```python
from build123d import *

# Parameters (mm, degrees)
BOSS_EXTRUDE1_DEPTH       = 3.175
SKETCH3_R                 = 5.55625
CUT_EXTRUDE1_DEPTH        = 31.120694713
SKETCH4_W                 = 31.75
SKETCH4_H                 = 3.175
BOSS_EXTRUDE2_DEPTH       = 12.7
SKETCH5_R                 = 1.5875
CUT_EXTRUDE2_DEPTH        = 45.22263278
F_2_0MM_DOWEL_HOLE1_D     = 2
F_2_0MM_DOWEL_HOLE1_DEPTH = 12.7
F_2_0MM_DOWEL_HOLE1_TIP   = 0.600860619


with BuildPart() as part:
    # Sketch1 → Boss-Extrude1 (new body)
    with BuildSketch(Plane.XY):
        with BuildLine():
            ThreePointArc((15.875, 0), (0, 15.875), (-15.875, 0))
            Line((-15.875, 0), (15.875, 0))
        make_face()
        with BuildLine():
            ThreePointArc((15.875, 0), (0, -15.875), (-15.875, 0))
            Line((-15.875, 0), (-15.875, -25.4))
            Line((-15.875, -25.4), (15.875, -25.4))
            Line((15.875, -25.4), (15.875, 0))
        make_face()
        with BuildLine():
            Line((15.875, 0), (-15.875, 0))
            ThreePointArc((-15.875, 0), (0, -15.875), (15.875, 0))
        make_face()
    extrude(amount=BOSS_EXTRUDE1_DEPTH)

    # Sketch3 → Cut-Extrude1 (cut, through all)
    with BuildSketch(Plane.XY.offset(3.175)):
        Circle(SKETCH3_R)
    extrude(amount=-CUT_EXTRUDE1_DEPTH, mode=Mode.SUBTRACT)

    # Sketch4 → Boss-Extrude2 (add)
    with BuildSketch(Plane.XY.offset(3.175)):
        with Locations((0, -23.8125)):
            Rectangle(SKETCH4_W, SKETCH4_H)
    extrude(amount=BOSS_EXTRUDE2_DEPTH)

    # Sketch5 → Cut-Extrude2 (cut, through all)
    with BuildSketch(Plane(origin=(0, -22.225, 0), x_dir=(1, 0, 0), z_dir=(0, 1, 0))):
        with Locations(Location((-9.525, -9.525, 0), (0, 0, 270))):
            Circle(SKETCH5_R)
        with Locations(Location((9.525, -9.525, 0), (0, 0, 90))):
            Circle(SKETCH5_R)
    extrude(amount=-CUT_EXTRUDE2_DEPTH, mode=Mode.SUBTRACT)

    # Ø2.0mm Dowel Hole1
    with Locations(Plane.XY.offset(3.175)):
        with Locations((-8.001, 0), (8.001, 0)):
            Hole(F_2_0MM_DOWEL_HOLE1_D / 2, depth=F_2_0MM_DOWEL_HOLE1_DEPTH)
            with Locations((0, 0, -(F_2_0MM_DOWEL_HOLE1_DEPTH + F_2_0MM_DOWEL_HOLE1_TIP / 2))):  # 118° drill point
                Cone(0, F_2_0MM_DOWEL_HOLE1_D / 2, F_2_0MM_DOWEL_HOLE1_TIP, mode=Mode.SUBTRACT)


solid = part.part
```
Here's how the part is built. I have some questions about the finished solid (model axes, mm). A direction names the side the tool comes from. Coordinates: 2 decimals unless noted, no trailing zeros. Order: outer loops, then holes, each group sorted by start corner. A loop starts at its lowest first (then second) coordinate and runs counter-clockwise, first axis right, second up.
Item 1: I need wall thicknesses on probe 1 along Y at (x, z) = (3, 5.5) (3 decimals); probe 2 along Z at (x, y) = (5, -6) (3 decimals); probe 3 along Y at (x, z) = (0.5, 2). Which ranges of each line are inside material? Lowest first, please.
Response values:
probe 1: y = -25.4 to -22.225
probe 2: z = 0 to 3.175
probe 3: y = -25.4 to -5.53, 5.53 to 15.87
Item 2: Which directions (+Z, -Z, +X, -X, +Y, -Y) give clear straight access to the entire face, cutting with the end or side of a thin tool? Please do faces 4 (the face through (0, -22.225, 9)), 5 (the face through (15.875, -16, 3)).
Response values:
face 4: +Z, +X, -X, +Y
face 5: +Z, -Z, +X, +Y, -Y
Item 3: Thinking about a two-plate mould opening in Y: for faces 1 (the face through (0, -25.4, 8)), 2 (the face through (8.8, -0.6, 1.6)), 3 (the face through (0, -24, 15.875)), which applies, pulls with the +Y half, pulls with the -Y half, needs draft (parallel to the pull), parting line crosses it, or undercut?
Response values:
face 1: pulls with the -Y half
face 2: undercut
face 3: needs draft
Item 4: If we section it at D-D, the plane y = 4: List the corners of the cut face in (x, z) for me (3 decimals), then the cut area to 3 significant figures.
Response values:
outline: (-15.363, 0) - (-3.856, 0) - (-3.856, 3.175) - (-15.363, 3.175) - close; (3.856, 0) - (15.363, 0) - (15.363, 3.175) - (3.856, 3.175) - close
area: 73.1 mm2
Item 5: I'm going to push flat-ended pins straight in: pin 1 Ø1.9 at (x, z) = (9.525, 9.525) entering from +Y; pin 2 Ø16 at (x, y) = (7.5, 2) entering from +Z (3 decimals); pin 3 Ø1.5 at (x, z) = (11, 11) entering from +Y (3 decimals); pin 4 Ø8 at (y, z) = (10, 2) entering from +X. Where does each tip first touch, or does it pass through?
Response values:
pin 1: passes through
pin 2: stops at z = 3.175
pin 3: stops at y = -22.225
pin 4: stops at x = 14.7
Item 6: If we section it at C-C, the plane y = -0.5: List the corners of the cut face in (x, z) for me (3 decimals).
Response values:
outline: (-15.875, 0) - (-8.867, 0) - (-8.867, 3.175) - (-15.875, 3.175) - close; (-7.135, 0) - (-5.534, 0) - (-5.534, 3.175) - (-7.135, 3.175) - close; (5.534, 0) - (7.135, 0) - (7.135, 3.175) - (5.534, 3.175) - close; (8.867, 0) - (15.875, 0) - (15.875, 3.175) - (8.867, 3.175) - close
Item 7: If we section it at A-A, the plane x = 0: List the corners of the cut face in (y, z) for me (3 decimals), then the cut area to 3 significant figures.
Response values:
outline: (-25.4, 0) - (-5.556, 0) - (-5.556, 3.175) - (-22.225, 3.175) - (-22.225, 15.875) - (-25.4, 15.875) - close; (5.556, 0) - (15.875, 0) - (15.875, 3.175) - (5.556, 3.175) - close
area: 136 mm2
Item 8: If we section it at B-B, the plane z = 1.25: Give the number of separate pieces and of enclosed holes in the cut face, then the cut area to 3 significant figures.
Response values:
separate pieces: 1
enclosed holes: 3
area: 1,100 mm2
